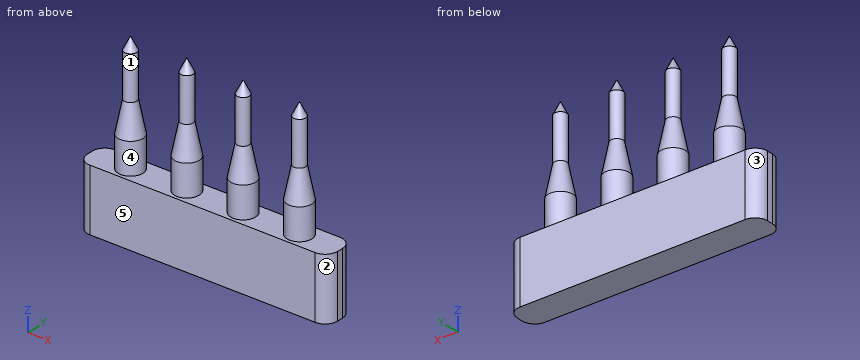
from build123d import *

# Parameters (mm, degrees)
F0_W     = 40
F0_H     = 5
F0_R     = 2
F0_R_2   = 1
F1_DEPTH = 10
F3_DEPTH = 5
F8_R     = 2


# Not quite as in the source:
# - a feature names something its author has since deleted; it is built from what else it names


with BuildPart() as f1:
    # F0 (on Top) → F1 (new body)
    with BuildSketch(Plane.XY):
        Rectangle(F0_W, F0_H)
        with Locations((-13.5, 0)):
            Circle(F0_R, mode=Mode.SUBTRACT)
        with BuildLine():
            ThreePointArc((-6.5, 0), (-4.5, 2), (-2.5, 0))
            ThreePointArc((-2.5, 0), (-4.5, -2), (-6.5, 0))
        make_face(mode=Mode.SUBTRACT)
        with BuildLine():
            ThreePointArc((6.5, 0), (4.5, -2), (2.5, 0))
            ThreePointArc((2.5, 0), (4.5, 2), (6.5, 0))
        make_face(mode=Mode.SUBTRACT)
        with BuildLine():
            ThreePointArc((15.5, 0), (13.5, -2), (11.5, 0))
            ThreePointArc((11.5, 0), (13.5, 2), (15.5, 0))
        make_face(mode=Mode.SUBTRACT)
        with BuildLine():
            ThreePointArc((15.5, 0), (13.5, 2), (11.5, 0))
            ThreePointArc((11.5, 0), (13.5, -2), (15.5, 0))
        make_face()
        with BuildLine():
            ThreePointArc((14.5, 0), (13.5, -1), (12.5, 0))
            ThreePointArc((12.5, 0), (13.5, 1), (14.5, 0))
        make_face(mode=Mode.SUBTRACT)
        with Locations((-13.5, 0)):
            Circle(F0_R)
        with Locations((-13.5, 0)):
            Circle(F0_R_2, mode=Mode.SUBTRACT)
        with BuildLine():
            ThreePointArc((14.5, 0), (13.5, 1), (12.5, 0))
            ThreePointArc((12.5, 0), (13.5, -1), (14.5, 0))
        make_face()
        with BuildLine():
            Line((4.5, 0), (3.5, 0))
            ThreePointArc((3.5, 0), (4.5, -1), (5.5, 0))
            Line((5.5, 0), (4.5, 0))
        make_face()
        with BuildLine():
            ThreePointArc((-5.5, 0), (-4.5, -1), (-3.5, 0))
            Line((-3.5, 0), (-4.5, 0))
            Line((-4.5, 0), (-5.5, 0))
        make_face()
        with Locations((-13.5, 0)):
            Circle(F0_R_2)
        with BuildLine():
            Line((-4.5, 0), (-3.5, 0))
            ThreePointArc((-3.5, 0), (-4.5, 1), (-5.5, 0))
            Line((-5.5, 0), (-4.5, 0))
        make_face()
        with BuildLine():
            ThreePointArc((5.5, 0), (4.5, 1), (3.5, 0))
            Line((3.5, 0), (4.5, 0))
            Line((4.5, 0), (5.5, 0))
        make_face()
        with BuildLine():
            ThreePointArc((-6.5, 0), (-4.5, -2), (-2.5, 0))
            Line((-2.5, 0), (-3.5, 0))
            ThreePointArc((-3.5, 0), (-4.5, -1), (-5.5, 0))
            Line((-5.5, 0), (-6.5, 0))
        make_face()
        with BuildLine():
            Line((3.5, 0), (2.5, 0))
            ThreePointArc((2.5, 0), (4.5, -2), (6.5, 0))
            Line((6.5, 0), (5.5, 0))
            ThreePointArc((5.5, 0), (4.5, -1), (3.5, 0))
        make_face()
        with BuildLine():
            ThreePointArc((6.5, 0), (4.5, 2), (2.5, 0))
            Line((2.5, 0), (3.5, 0))
            ThreePointArc((3.5, 0), (4.5, 1), (5.5, 0))
            Line((5.5, 0), (6.5, 0))
        make_face()
        with BuildLine():
            Line((-3.5, 0), (-2.5, 0))
            ThreePointArc((-2.5, 0), (-4.5, 2), (-6.5, 0))
            Line((-6.5, 0), (-5.5, 0))
            ThreePointArc((-5.5, 0), (-4.5, 1), (-3.5, 0))
        make_face()
    extrude(amount=-F1_DEPTH)

    # F0 (on Top) → F3 (join)
    with BuildSketch(Plane.XY):
        with Locations((-13.5, 0)):
            Circle(F0_R)
        with Locations((-13.5, 0)):
            Circle(F0_R_2, mode=Mode.SUBTRACT)
        with BuildLine():
            ThreePointArc((15.5, 0), (13.5, 2), (11.5, 0))
            ThreePointArc((11.5, 0), (13.5, -2), (15.5, 0))
        make_face()
        with BuildLine():
            ThreePointArc((14.5, 0), (13.5, -1), (12.5, 0))
            ThreePointArc((12.5, 0), (13.5, 1), (14.5, 0))
        make_face(mode=Mode.SUBTRACT)
        with BuildLine():
            Line((4.5, 0), (3.5, 0))
            ThreePointArc((3.5, 0), (4.5, -1), (5.5, 0))
            Line((5.5, 0), (4.5, 0))
        make_face()
        with BuildLine():
            ThreePointArc((14.5, 0), (13.5, 1), (12.5, 0))
            ThreePointArc((12.5, 0), (13.5, -1), (14.5, 0))
        make_face()
        with BuildLine():
            ThreePointArc((5.5, 0), (4.5, 1), (3.5, 0))
            Line((3.5, 0), (4.5, 0))
            Line((4.5, 0), (5.5, 0))
        make_face()
        with BuildLine():
            ThreePointArc((-5.5, 0), (-4.5, -1), (-3.5, 0))
            Line((-3.5, 0), (-4.5, 0))
            Line((-4.5, 0), (-5.5, 0))
        make_face()
        with BuildLine():
            Line((-4.5, 0), (-3.5, 0))
            ThreePointArc((-3.5, 0), (-4.5, 1), (-5.5, 0))
            Line((-5.5, 0), (-4.5, 0))
        make_face()
        with Locations((-13.5, 0)):
            Circle(F0_R_2)
        with BuildLine():
            ThreePointArc((-6.5, 0), (-4.5, -2), (-2.5, 0))
            Line((-2.5, 0), (-3.5, 0))
            ThreePointArc((-3.5, 0), (-4.5, -1), (-5.5, 0))
            Line((-5.5, 0), (-6.5, 0))
        make_face()
        with BuildLine():
            Line((-3.5, 0), (-2.5, 0))
            ThreePointArc((-2.5, 0), (-4.5, 2), (-6.5, 0))
            Line((-6.5, 0), (-5.5, 0))
            ThreePointArc((-5.5, 0), (-4.5, 1), (-3.5, 0))
        make_face()
        with BuildLine():
            ThreePointArc((6.5, 0), (4.5, 2), (2.5, 0))
            Line((2.5, 0), (3.5, 0))
            ThreePointArc((3.5, 0), (4.5, 1), (5.5, 0))
            Line((5.5, 0), (6.5, 0))
        make_face()
        with BuildLine():
            Line((3.5, 0), (2.5, 0))
            ThreePointArc((2.5, 0), (4.5, -2), (6.5, 0))
            Line((6.5, 0), (5.5, 0))
            ThreePointArc((5.5, 0), (4.5, -1), (3.5, 0))
        make_face()
    extrude(amount=F3_DEPTH)

    # F2 (on Front) → F4 (revolve)
    with BuildSketch(Plane.XZ):
        Polygon((-13.5, 19), (-13.5, 10), (-12.5, 10), (-12.5, 17), align=None)
        Polygon((-13.5, 10), (-13.5, 5), (-11.5, 5), (-12.5, 10), align=None)
    revolve(axis=Axis((-13.5, 0, 14.5), (0, 0, 1)))

    # F2 (on Front) → F5 (revolve)
    with BuildSketch(Plane.XZ):
        Polygon((-4.5, 19), (-4.5, 10), (-3.5, 10), (-3.5, 17), align=None)
        Polygon((-4.5, 10), (-4.5, 5), (-2.5, 5), (-3.5, 10), align=None)
    revolve(axis=Axis((-4.5, 0, 14.5), (0, 0, 1)))

    # F2 (on Front) → F6 (revolve)
    with BuildSketch(Plane.XZ):
        Polygon((2.5, 5), (4.5, 5), (4.5, 10), (3.5, 10), align=None)
        Polygon((3.5, 10), (4.5, 10), (4.5, 19), (3.5, 17), align=None)
    revolve(axis=Axis((4.5, 0, 14.5), (0, 0, 1)))

    # F2 (on Front) → F7 (revolve)
    with BuildSketch(Plane.XZ):
        Polygon((13.5, 5), (13.5, 10), (13.5, 19), (12.5, 17), (12.5, 10), (11.5, 5), align=None)
    revolve(axis=Axis((13.5, 0, 14.5), (0, 0, 1)))

    # F8
    f8_edges = [f1.edges().sort_by_distance(p)[0] for p in [
        (-20, -2.5, -5),
        (-20, 2.5, -5),
        (20, -2.5, -5),
        (20, 2.5, -5),
    ]]
    fillet(f8_edges, radius=F8_R)


solid = f1.part
Part model, mm, in its own coordinate system. Face numbers are marked on the shaded views. A direction names the side the tool comes from. Give positions to 0.01 mm unless a question says otherwise; leave off trailing zeros. Loops run counter-clockwise (first coordinate to the right, second up) from the corner with the lowest first, then second, coordinate; pieces in that order, holes last. Notation, with made-up numbers: M -32,46.25 L 10,46.25 A25 ccw 10,80.25 Z; hole C -36.75,45 d6. An arc over 180 degrees is marked long. Put each result on its own line as item: value. Start each with the question number.
1) 3-axis set-ups, long thin cutter, end or side, ignore diameter. For the marked faces 4 and 5: which of +Z, -Z, +X, -X, +Y, -Y reach the whole face in a straight line?
2) Saw through at C-C (x = -7). List the corners of the cut face in (y, z), then the cut area to 3 significant figures.
3) Saw through at A-A (z = -7). List the corners of the cut face in (x, y), then the cut area to 3 significant figures.
4) Probe probe 1 along X at (y, z) = (-0.55, 11); probe 2 along X at (y, z) = (1.7, 2); probe 3 along Z at (x, y) = (7, -0.1). List the from-to ranges inside material, lowest first.
5) Saw through at B-B (z = 7.5). List the corners of the cut face in (x, y).
6) Flat gauge pins, fed straight in: pin 1 (4 mm diameter, centred on x = -4.5, z = 15.5, fed in from +Y); pin 2 (1.5 mm diameter, centred on x = -1, z = 5, fed in from +Y). Where does each tip first touch, or does it go through?
7) Pull direction X, two halves, no side cores. Call the marked faces 1, 2 and 3: +X half, -X half, draft (parallel to the pull), parting line (faces both ways), or undercut.
Numbers:
1. face 4: +Z
1. face 5: +Z, -Z, +X, -X, -Y
2. outline: M -2.5,-10 L 2.5,-10 L 2.5,0 L -2.5,0 Z
2. area: 50.0 mm^2
3. outline: M -20,-0.5 A2 ccw -18,-2.5 L 18,-2.5 A2 ccw 20,-0.5 L 20,0.5 A2 ccw 18,2.5 L -18,2.5 A2 ccw -20,0.5 Z
3. area: 197 mm^2
4. probe 1: -14.34 to -12.66, -5.34 to -3.66, 3.66 to 5.34, 12.66 to 14.34
4. probe 2: -14.55 to -12.45, -5.55 to -3.45, 3.45 to 5.55, 12.45 to 14.55
4. probe 3: -10 to 0
5. outline: C -13.5,0 d3; C -4.5,0 d3; C 4.5,0 d3; C 13.5,0 d3
6. pin 1: y = 1
6. pin 2: through
7. face 1: undercut
7. face 2: +X half
7. face 3: -X half
